Design review of the part built by this model. Coordinates are the model's own, in mm. A direction names the side the tool comes from. Give positions to 0.01 mm unless a question says otherwise; leave off trailing zeros. Loops run counter-clockwise (first coordinate to the right, second up) from the corner with the lowest first, then second, coordinate; pieces in that order, holes last. Notation, with made-up numbers: (7.25, 80) - (25.25, 80) arc R27 ccw to (25.25, 113) - close; hole circle Ø1 at (-7.75, 64.5). An arc over 180 degrees is marked (long way). One line per item, written item: value. Start each with the question number.
Autodesk Inventor part; units mm, degrees
ref_plane "YZ Plane" through (0, 0, 0) normal (1, 0, 0) x (0, 1, 0)
ref_plane "XZ Plane" through (0, 0, 0) normal (0, 1, 0) x (-1, 0, 0)
ref_plane "XY Plane" through (0, 0, 0) normal (0, 0, 1) x (1, 0, 0)
sketch "Sketch1" plane through (0, 0, 0) normal (1, 0, 0) x (0, 1, 0)
  line L0 (48.5, 0) -> (52.5, 0)
  line L1 (52.5, 0) -> (52.5, 8)
  line L2 (-4, 8) -> (-4, 0)
  line L3 (-4, 0) -> (0, 0)
  line L4 (0, 0) -> (0, 6)
  line L5 (4.5, 10.5) -> (44, 10.5)
  line L6 (48.5, 6) -> (48.5, 0)
  line L7 (3.5, 15.5) -> (45, 15.5)
  line L8 (45, 15.5) -> (52.5, 8)
  line L9 (-4, 8) -> (3.5, 15.5)
  line L10 (48.5, 6) -> (45, 6)
  line L11 (45, 6) -> (45, 9.5)
  line L12 (0, 6) -> (3.5, 6)
  line L13 (3.5, 6) -> (3.5, 9.5)
  arc A0 (45, 9.5) -> (44, 10.5) centre (44, 9.5) ccw
  arc A1 (4.5, 10.5) -> (3.5, 9.5) centre (4.5, 9.5) ccw
  point P0 (0, 0)
  point P1 (24.25, 15.5)
  point P2 (24.25, 10.5)
  dimension "d4" = 48.5
  dimension "d31" = 5
  dimension "d37" = 4
  dimension "d46" = 3.5
  dimension "d48" = 1
  dimension "d50" = 8
  dimension "d51" = 4.5
  dimension "d52" = 6
extrude "Extrusion1" add sketch "Sketch1" along normal blind 6
fillet "Fillet1" radius 5 4 edges at (3, 3.5, 15.5) (3, 45, 15.5) (3, 52.5, 8) (3, -4, 8)
equation "\"d4\" = ServoMount"
equation "\"ServoMountLength\" = 48.5"
properties part number "27080914ServoMount"
(1) For pin 1 Ø1.8 at (x, y) = (3.5, 47) entering from -Z; pin 2 Ø1 at (x, z) = (3, 7.5) entering from +Y; pin 3 Ø1.8 at (x, z) = (1.5, 7.5) entering from -Y, all flat-tipped, find the tip position at first contact; note any pin that passes through.
(2) Draft analysis for pull direction Y (two halves, no side actions). For faces 3 (the flat face through (3, 48.7, 11.8)), 4 (the flat face through (3, 0, 3)), 5 (the cylindrical face through (3.04, -3.61, 7.87)), 6 (the flat face through (3, -2, 0)), state which applies: pulls with the +Y half, pulls with the -Y half, needs draft (parallel to the pull), parting line crosses it, or undercut.
(3) Take a section at C-C on y = 33. State the section outline as (x, z) points.
(4) Machinability: for faces 1 (the flat face through (3, 3.5, 8)), 2 (the flat face through (3, 50, 0)), which of the approach directions +Z, -Z, +X, -X, +Y, -Y give a long, thin tool a straight path to every point of the face, cutting with its end or side? Answer none if there is none.
(5) To check wall thickness, follow L1, parallel to Y at x = 1.6, z = 1.25; L2, parallel to Z at x = 3.45, y = 15.5; L3, parallel to Y at x = 4.55, z = 8.5. State the ranges of each line that lie inside material, in increasing order. Write a range as from..to.
(6) Take a section at A-A on z = 2.5. State the section outline as (x, y) points, and give its area (3 significant figures).
(7) Take a section at D-D on z = 8. State the section outline as (x, y) points.
(8) Take a section at B-B on x = 4.2. State the section outline as (y, z) points.
Here are the results:
1. pin 1: z = 6
1. pin 2: y = 52.38
1. pin 3: y = -3.95
2. face 3: pulls with the +Y half
2. face 4: undercut
2. face 5: pulls with the -Y half
2. face 6: needs draft
3. outline: (0, 10.5) - (6, 10.5) - (6, 15.5) - (0, 15.5) - close
4. face 1: -Z, +X, -X
4. face 2: -Z, +X, -X, +Y, -Y
5. L1: -4..0, 48.5..52.5
5. L2: 10.5..15.5
5. L3: -3.29..3.5, 45..51.79
6. outline: (0, -4) - (6, -4) - (6, 0) - (0, 0) - close; (0, 48.5) - (6, 48.5) - (6, 52.5) - (0, 52.5) - close
6. area: 48.0 mm²
7. outline: (0, -3.55) - (6, -3.55) - (6, 3.5) - (0, 3.5) - close; (0, 45) - (6, 45) - (6, 52.05) - (0, 52.05) - close
8. outline: (-4, 0) - (0, 0) - (0, 6) - (3.5, 6) - (3.5, 9.5) arc R1 cw to (4.5, 10.5) - (44, 10.5) arc R1 cw to (45, 9.5) - (45, 6) - (48.5, 6) - (48.5, 0) - (52.5, 0) - (52.5, 5.93) arc R5 ccw to (51.04, 9.46) - (46.46, 14.04) arc R5 ccw to (42.93, 15.5) - (5.57, 15.5) arc R5 ccw to (2.04, 14.04) - (-2.54, 9.46) arc R5 ccw to (-4, 5.93) - close
